Verification items for the finished model (mm, model axes). Round coordinates to 2 decimals unless told otherwise and drop trailing zeros. Write each loop counter-clockwise with the first axis right and the second up, starting at its lowest first coordinate (ties: lowest second). Pieces come first, ordered by that corner, then holes. Notation, with made-up numbers: (17.5, 69) - (28.5, 69) arc R17 cw to (28.5, 97) - close; hole circle Ø10 at (46.5, -3). An arc over 180 degrees is marked (long way). Answer as a JSON object with one key per item and string values. Group by question number.
1) Go/stop test with flat-tipped pins: pin 1 Ø2 at (y, z) = (-7.5, 2.5) entering from -X; pin 2 Ø1.5 at (y, z) = (2, 3) entering from -X; pin 3 Ø6.5 at (x, y) = (-75, -15) entering from -Z; pin 4 Ø3.5 at (x, y) = (75, 15) entering from -Z. Record where each tip stops, or that it passes through.
2) Section check A-A (y = 0). Enter the section's corners in (x, z), then the cut area to 3 significant figures.
3) Section check C-C (x = -75). Enter the section's corners in (y, z).
4) Section check D-D (z = 4.4). Enter the section's corners in (x, y).
5) Section check B-B (x = -10.5). Enter the section's corners in (y, z), then the cut area to 3 significant figures.
6) Thickness scan on line 1 (Y direction, x = 75, z = 1.8); line 2 (Y direction, x = -38.5, z = 0.85); line 3 (X direction, y = -5, z = 4.8). Record the ranges inside material, lowest first.
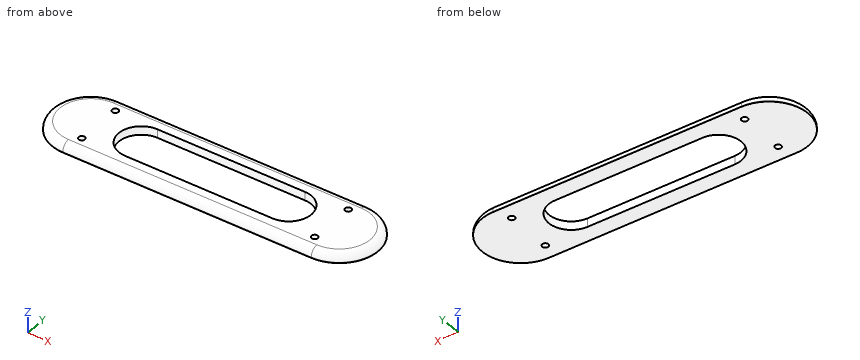
```python
from build123d import *

# Parameters (mm, degrees)
SKETCH1_R           = 2
BOSS_EXTRUDE2_DEPTH = 5.5
FILLET1_R           = 5


with BuildPart() as part:
    # Sketch1 → Boss-Extrude2 (new body)
    with BuildSketch(Plane.XY):
        with BuildLine():
            Line((-80, -25), (80, -25))
            ThreePointArc((80, -25), (105, 0), (80, 25))
            Line((80, 25), (-80, 25))
            ThreePointArc((-80, 25), (-105, 0), (-80, -25))
        make_face()
        with Locations((-75, 15)):
            Circle(SKETCH1_R, mode=Mode.SUBTRACT)
        with Locations(Location((-75, -15, 0), (0, 0, 180))):
            Circle(SKETCH1_R, mode=Mode.SUBTRACT)
        with Locations((75, -15)):
            Circle(SKETCH1_R, mode=Mode.SUBTRACT)
        with Locations(Location((75, 15, 0), (0, 0, 180))):
            Circle(SKETCH1_R, mode=Mode.SUBTRACT)
        with BuildLine():
            Line((-47.5, 14.5), (47.5, 14.5))
            ThreePointArc((47.5, 14.5), (62, 0), (47.5, -14.5))
            Line((47.5, -14.5), (-47.5, -14.5))
            ThreePointArc((-47.5, -14.5), (-62, 0), (-47.5, 14.5))
        make_face(mode=Mode.SUBTRACT)
    extrude(amount=BOSS_EXTRUDE2_DEPTH)

    # Fillet1
    fillet1_edges = [part.edges().sort_by_distance(p)[0] for p in [
        (105, 0, 5.5),
        (0, 25, 5.5),
        (-105, 0, 5.5),
        (0, -25, 5.5),
    ]]
    fillet(fillet1_edges, radius=FILLET1_R)


solid = part.part
```
Returned:
{
 "1": {"pin 1": "x = -103.88", "pin 2": "x = -104.61", "pin 3": "z = 0", "pin 4": "through"},
 "2": {"outline": "(-105, 0) - (-62, 0) - (-62, 5.5) - (-100, 5.5) arc R5 ccw to (-105, 0.5) - close; (62, 0) - (105, 0) - (105, 0.5) arc R5 ccw to (100, 5.5) - (62, 5.5) - close", "area": "462 mm2"},
 "3": {"outline": "(-25, 0) - (-17, 0) - (-17, 5.5) - (-20, 5.5) arc R5 ccw to (-25, 0.5) - close; (-13, 0) - (13, 0) - (13, 5.5) - (-13, 5.5) - close; (17, 0) - (25, 0) - (25, 0.5) arc R5 ccw to (20, 5.5) - (17, 5.5) - close"},
 "4": {"outline": "(-80, -23.13) - (80, -23.13) arc R23.13 ccw to (80, 23.13) - (-80, 23.13) arc R23.13 ccw to start; hole circle Ø4 at (-75, -15); hole circle Ø4 at (-75, 15); hole (-47.5, -14.5) - (47.5, -14.5) arc R14.5 ccw to (47.5, 14.5) - (-47.5, 14.5) arc R14.5 ccw to start; hole circle Ø4 at (75, -15); hole circle Ø4 at (75, 15)"},
 "5": {"outline": "(-25, 0) - (-14.5, 0) - (-14.5, 5.5) - (-20, 5.5) arc R5 ccw to (-25, 0.5) - close; (14.5, 0) - (25, 0) - (25, 0.5) arc R5 ccw to (20, 5.5) - (14.5, 5.5) - close", "area": "105 mm2"},
 "6": {"line 1": "-24.83 to -17, -13 to 13, 17 to 24.83", "line 2": "-24.99 to -14.5, 14.5 to 24.99", "line 3": "-101.99 to -61.11, 61.11 to 101.99"}
}
